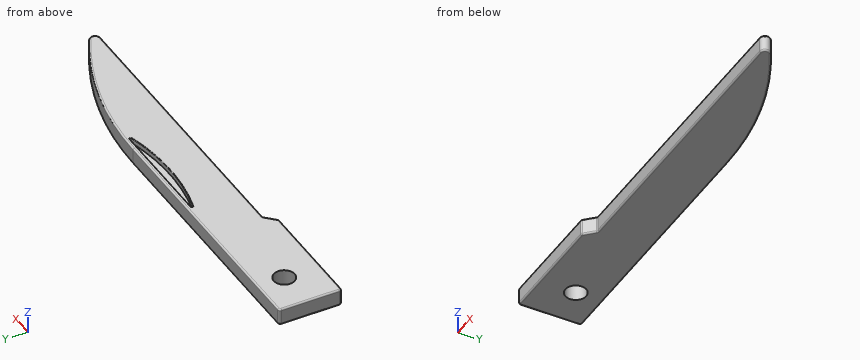
from build123d import *

# Parameters (mm, degrees)
BOSS_EXTRUDE1_DEPTH = 1.6
FILLET1_R           = 0.5
FILLET2_R           = 0.25
FILLET3_R           = 0.15
SKETCH2_R           = 1
CUT_EXTRUDE1_DEPTH  = 42.21969505
CUT_EXTRUDE2_DEPTH  = 0.5
FILLET4_R           = 0.1
FILLET5_R           = 0.05


with BuildPart() as part:
    # Sketch1 → Boss-Extrude1 (new body)
    with BuildSketch(Plane.XY):
        with BuildLine():
            Line((0, 0), (0, 6))
            Line((0, 6), (25.416876048, 6))
            ThreePointArc((25.416876048, 6), (34.077130086, 4.722813233), (42, 1))
            Line((42, 1), (12, 1))
            Line((12, 1), (11, 0))
            Line((11, 0), (0, 0))
        make_face()
    extrude(amount=BOSS_EXTRUDE1_DEPTH)

    # Fillet1
    fillet1_edges = [part.edges().sort_by_distance(p)[0] for p in [
        (42, 1, 0.8),
    ]]
    fillet(fillet1_edges, radius=FILLET1_R)

    # Fillet2
    fillet2_edges = [part.edges().sort_by_distance(p)[0] for p in [
        (0, 0, 0.8),
        (0, 6, 0.8),
        (12, 1, 0.8),
        (11, 0, 0.8),
    ]]
    fillet(fillet2_edges, radius=FILLET2_R)

    # Fillet3
    fillet3_edges = [part.edges().sort_by_distance(p)[0] for p in [
        (33.228210707, 4.96520414, 0),
        (33.228210707, 4.96520414, 1.6),
        (12.833438024, 6, 1.6),
        (40.732026425, 1.369811089, 0),
        (40.732026425, 1.369811089, 1.6),
        (0, 3, 0),
        (0, 3, 1.6),
        (26.176413207, 1, 0),
        (11.5, 0.5, 0),
        (5.573223305, 0, 0),
        (0.073223305, 0.073223305, 0),
        (10.992117467, 0.019030117, 0),
        (0.073223305, 5.926776695, 0),
        (26.176413207, 1, 1.6),
        (5.573223305, 0, 1.6),
        (11.5, 0.5, 1.6),
        (0.073223305, 0.073223305, 1.6),
        (10.992117467, 0.019030117, 1.6),
        (0.073223305, 5.926776695, 1.6),
        (12.007882533, 0.980969883, 0),
        (12.007882533, 0.980969883, 1.6),
        (12.833438024, 6, 0),
    ]]
    fillet(fillet3_edges, radius=FILLET3_R)

    # Sketch2 → Cut-Extrude1 (cut, through all)
    with BuildSketch(Plane.XY.offset(1.6)):
        with Locations((3.75, 3.45)):
            Circle(SKETCH2_R)
    extrude(amount=-CUT_EXTRUDE1_DEPTH, mode=Mode.SUBTRACT)

    # Sketch3 → Cut-Extrude2 (cut)
    with BuildSketch(Plane.XY.offset(1.6)):
        with BuildLine():
            Line((15.416876048, 5.6), (27.416876048, 5.6))
            ThreePointArc((27.416876048, 5.6), (21.416876048, 4.678784028), (15.416876048, 5.6))
        make_face()
    extrude(amount=-CUT_EXTRUDE2_DEPTH, mode=Mode.SUBTRACT)

    # Fillet4
    fillet4_edges = [part.edges().sort_by_distance(p)[0] for p in [
        (27.416876048, 5.6, 1.35),
        (15.416876048, 5.6, 1.35),
    ]]
    fillet(fillet4_edges, radius=FILLET4_R)

    # Fillet5
    fillet5_edges = [part.edges().sort_by_distance(p)[0] for p in [
        (21.416876048, 5.6, 1.6),
        (21.416876048, 4.678784028, 1.6),
        (26.824849278, 5.513461428, 1.6),
        (16.008902818, 5.513461428, 1.6),
    ]]
    fillet(fillet5_edges, radius=FILLET5_R)


solid = part.part
Source: CAD feature listing. Evaluate the final solid. Frame: model axes, mm. Round coordinates to 2 decimals unless told otherwise and drop trailing zeros. Loops run counter-clockwise (first coordinate to the right, second up) from the corner with the lowest first, then second, coordinate; pieces in that order, holes last. Notation, with made-up numbers: M 63.5,14 L 102.5,14 A31 cw 102.5,50 Z; hole C 8.25,23 d10. An arc over 180 degrees is marked long. Return JSON: item names as keys, results as strings. Group by question number.
1. Section query B-B on x = 3.75. Output: boundary loops of the cut face in (y, z), and give its area (3 significant figures).
2. Section query A-A on z = 0.8. Output: boundary loops of the cut face in (x, y).
3. Material intervals for line 1 along Y through (x, z) = (3.75, 0.5); line 2 along Y through (x, z) = (20, 0.85); line 3 along X through (y, z) = (2.75, 1.05), sorted ascending. Write a range as from..to.
Checks:
{
 "1": {"outline": "M 0,0.15 A0.15 ccw 0.15,0 L 2.45,0 L 2.45,1.6 L 0.15,1.6 A0.15 ccw 0,1.45 Z; M 4.45,0 L 5.85,0 A0.15 ccw 6,0.15 L 6,1.45 A0.15 ccw 5.85,1.6 L 4.45,1.6 Z", "area": "6.38 mm²"},
 "2": {"outline": "M 0,0.25 A0.25 ccw 0.25,0 L 10.9,0 A0.25 ccw 11.07,0.07 L 11.93,0.93 A0.25 cw 12.1,1 L 40.25,1 A0.5 ccw 40.5,1.93 A30 ccw 25.42,6 L 0.25,6 A0.25 ccw 0,5.75 Z; hole C 3.75,3.45 d2"},
 "3": {"line 1": "y = 0..2.45, 4.45..6", "line 2": "y = 1..6", "line 3": "x = 0..3.04, 4.46..39"}
}
